Read the model definition and answer for the solid it produces. Units are mm, in the model's axes. Face numbers are marked on the shaded views. A direction names the side the tool comes from. Coordinates: 2 decimals unless noted, no trailing zeros. Write each loop counter-clockwise with the first axis right and the second up, starting at its lowest first coordinate (ties: lowest second). Pieces come first, ordered by that corner, then holes.
(1) The part is cut by section C-C, the plane y = 2.6. Determine the outline of the cut face in (x, z), and give its area (3 significant figures).
(2) The part is cut by section A-A, the plane y = -1.6. Determine the outline of the cut face in (x, z).
(3) Determine the mould class of the marked faces 1, 2 and 3 for opening direction Z: pulls with the +Z half, pulls with the -Z half, needs draft (parallel to the pull), parting line crosses it, or undercut.
(4) Which of the six approach directions +Z, -Z, +X, -X, +Y, -Y give full straight-line access (tool end or side, diameter ignored) to the marked faces 4 and 5?
(5) Given pin 1 (2.5 mm diameter, centred on x = -0.5, z = 0.5, fed in from +Y); pin 2 (1 mm diameter, centred on y = 1.5, z = 1.5, fed in from -X), each flat-ended and moving along its own axis, determine where each tip first touches the part or whether it passes through.
(6) Straight lines are drawn through the part: line 1 along X through (y, z) = (1.6, -0.5) (3 decimals); line 2 along X through (y, z) = (1.95, -0.25); line 3 along Y through (x, z) = (0.75, -1). For each, find the intervals that lie inside material, in ascending order.
```python
from build123d import *

# Parameters (mm, degrees)
F0_R     = 4
F1_DEPTH = 2
F2_R     = 1.99999
F3_R     = 2.8
F4_DEPTH = 3.1
F5_R     = 1.5
F6_DEPTH = 3


# Not quite as in the source:
# - a fillet or chamfer is up to 0.001 mm smaller than in the source, because OpenCascade refuses the exact size


with BuildPart() as f1:
    # F0 (on Front) → F1 (new body)
    with BuildSketch(Plane.XZ):
        Circle(F0_R)
    extrude(amount=F1_DEPTH)

    # F2 (radius 2 in the source; OpenCascade refuses exactly that, so slightly less here)
    f2_edges = [f1.edges().sort_by_distance(p)[0] for p in [
        (-4, -2, 0),
    ]]
    fillet(f2_edges, radius=F2_R)

    # F3 (on face) → F4 (join)
    with BuildSketch(Plane(origin=(0, 0, 0), x_dir=(-1, 0, 0), z_dir=(0, 1, 0))):
        Circle(F3_R)
    extrude(amount=F4_DEPTH)

    # F5 (on face) → F6 (cut)
    with BuildSketch(Plane(origin=(0, 3.1, 0), x_dir=(-1, 0, 0), z_dir=(0, 1, 0))):
        with Locations((0.0365495689, 0.0300457796)):
            Circle(F5_R)
    extrude(amount=-F6_DEPTH, mode=Mode.SUBTRACT)


solid = f1.part
```
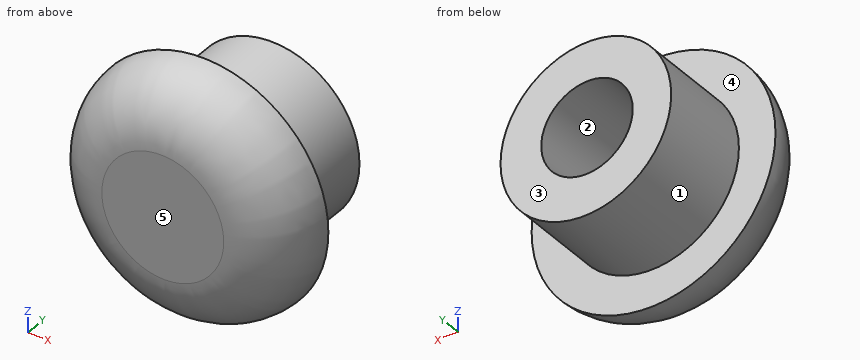
Computed:
1. outline: circle Ø5.6 at (0, 0); hole circle Ø3 at (-0.04, 0.03)
1. area: 17.6 mm2
2. outline: circle Ø6.4 at (0, 0)
3. face 1: parting line crosses it
3. face 2: undercut
3. face 3: needs draft
4. face 4: +Y
4. face 5: +Z, -Z, +X, -X, -Y
5. pin 1: stops at y = 3.1
5. pin 2: stops at x = -2.62
6. line 1: x = -2.755 to -1.44, 1.367 to 2.755
6. line 2: x = -2.79 to -1.51, 1.44 to 2.79
6. line 3: y = -2 to 0.1
